```python
from build123d import *

# Parameters (mm, degrees)
F0_W          = 400
F0_H          = 12
F1_DEPTH      = 700
F2_W          = 12
F2_H          = 50
F3_DEPTH      = 50
F4_R          = 3
F5_DEPTH      = 381.001
F5_DEPTH_BACK = 19.001


with BuildPart() as f1:
    # F0 (on Front) → F1 (new body)
    with BuildSketch(Plane.XZ):
        with Locations((200, 6)):
            Rectangle(F0_W, F0_H)
    extrude(amount=-F1_DEPTH)

    # F2 (on face) → F3 (join)
    with BuildSketch(Plane.XY.offset(12)):
        with Locations((25, 25)):
            Rectangle(F2_W, F2_H)
        with Locations((375, 25)):
            Rectangle(F2_W, F2_H)
        with Locations((6, 525)):
            Rectangle(F2_W, F2_H)
        with Locations((394, 525)):
            Rectangle(F2_W, F2_H)
    extrude(amount=F3_DEPTH)

    # F4 (on face) → F5 (cut, two sides)
    with BuildSketch(Plane(origin=(19, 0, 0), x_dir=(0, -1, 0), z_dir=(-1, 0, 0))) as f5_sk:
        with Locations((-25, 42)):
            Circle(F4_R)
        with Locations((-525, 42)):
            Circle(F4_R)
    extrude(amount=-F5_DEPTH, mode=Mode.SUBTRACT)
    extrude(f5_sk.sketch, amount=F5_DEPTH_BACK, mode=Mode.SUBTRACT)


solid = f1.part
```
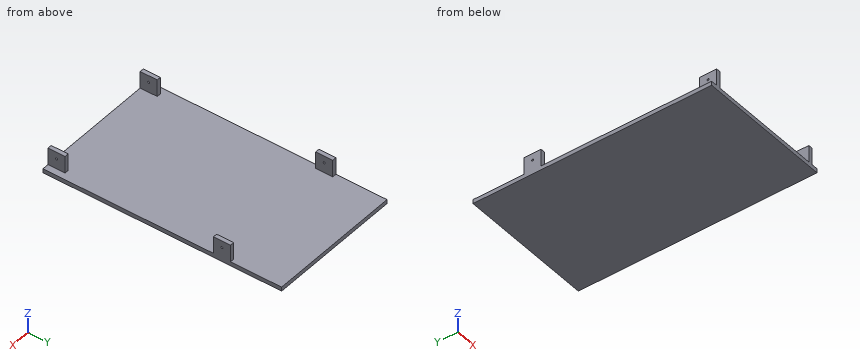
Geometry check sheet. Reference: the model listing, model coordinates, mm. Coordinates: 2 decimals unless noted, no trailing zeros. Order: outer loops, then holes, each group sorted by start corner. A loop starts at its lowest first (then second) coordinate and runs counter-clockwise, first axis right, second up. Notation, with made-up numbers: M 24.5,-29.5 L 57.5,-29.5 A26 cw 57.5,6.5 Z; hole C -29.5,39 d2. An arc over 180 degrees is marked long. Answer as a JSON object with one key per item and string values.
Q1. Scan lines: line 1 (Y direction, x = 4, z = 42); line 2 (Z direction, x = 6.75, y = 525); line 3 (Z direction, x = 155, y = 128.5). Record each from-to range of solid material in increasing order.
Results are:
{"line 1": "y = 500 to 522, 528 to 550", "line 2": "z = 0 to 39, 45 to 62", "line 3": "z = 0 to 12"}
Q2. Cross-section at A-A on z = 31. Record the cut outline in (x, y).
Results are:
{"outline": "M 0,500 L 12,500 L 12,550 L 0,550 Z; M 19,0 L 31,0 L 31,50 L 19,50 Z; M 369,0 L 381,0 L 381,50 L 369,50 Z; M 388,500 L 400,500 L 400,550 L 388,550 Z"}
Q3. Depth check by flat-ended pin: pin 1 Ø15 at (y, z) = (14, 30.5) entering from +X; pin 2 Ø3.5 at (x, z) = (392, 31.5) entering from +Y; pin 3 Ø4 at (x, y) = (292, 169) entering from +Z; pin 4 Ø5 at (y, z) = (525, 42) entering from +X. Enter the tip coordinate at first touch or a pass-through.
Results are:
{"pin 1": "stops at x = 381", "pin 2": "stops at y = 550", "pin 3": "stops at z = 12", "pin 4": "passes through"}
Q4. Cross-section at B-B on x = 249. Record the cut outline in (y, z), and give its area (3 significant figures).
Results are:
{"outline": "M 0,0 L 700,0 L 700,12 L 0,12 Z", "area": "8,400 mm²"}
Q5. Cross-section at C-C on y = 573. Record the cut outline in (x, z), and give its area (3 significant figures).
Results are:
{"outline": "M 0,0 L 400,0 L 400,12 L 0,12 Z", "area": "4,800 mm²"}
